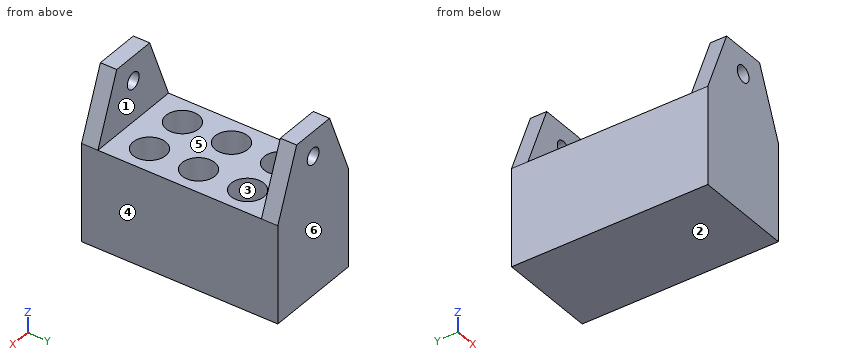
```python
from build123d import *

# Parameters (mm, degrees)
F0_W       = 38.1
F0_H       = 76.2
F0_R       = 6.35
F1_DEPTH   = 38.1
F2_DEPTH   = 12.7
F3_W       = 38.1
F3_H       = 6.35
F4_DEPTH   = 25.4
F5_SIZE2   = 10.16
F5_SIZE    = 25.4
F6_SIZE2   = 10.16
F6_SIZE    = 25.4
F6_2_SIZE2 = 10.16
F6_2_SIZE  = 25.4
F7_R       = 3.175
F8_DEPTH   = 105.84064


with BuildPart() as f1:
    # F0 (on Top) → F1 (new body)
    with BuildSketch(Plane.XY):
        with Locations((19.05, 38.1)):
            Rectangle(F0_W, F0_H)
        with Locations((10.16, 19.05)):
            Circle(F0_R, mode=Mode.SUBTRACT)
        with Locations((27.94, 19.05)):
            Circle(F0_R, mode=Mode.SUBTRACT)
        with Locations((10.16, 38.1)):
            Circle(F0_R, mode=Mode.SUBTRACT)
        with Locations((10.16, 57.15)):
            Circle(F0_R, mode=Mode.SUBTRACT)
        with Locations((27.94, 38.1)):
            Circle(F0_R, mode=Mode.SUBTRACT)
        with Locations((27.94, 57.15)):
            Circle(F0_R, mode=Mode.SUBTRACT)
    extrude(amount=F1_DEPTH)

    # F0 (on Top) → F2 (join)
    with BuildSketch(Plane.XY):
        with Locations((10.16, 57.15)):
            Circle(F0_R)
        with Locations((27.94, 57.15)):
            Circle(F0_R)
        with Locations((27.94, 38.1)):
            Circle(F0_R)
        with Locations((10.16, 19.05)):
            Circle(F0_R)
        with Locations((27.94, 19.05)):
            Circle(F0_R)
        with Locations((10.16, 38.1)):
            Circle(F0_R)
    extrude(amount=F2_DEPTH)

    # F3 (on face) → F4 (join)
    with BuildSketch(Plane.XY.offset(38.1)):
        with Locations((19.05, 73.025)):
            Rectangle(F3_W, F3_H)
        with Locations((19.05, 3.175)):
            Rectangle(F3_W, F3_H)
    extrude(amount=F4_DEPTH)

    # F5
    f5_edges = [f1.edges().sort_by_distance(p)[0] for p in [
        (38.1, 73.025, 63.5),
        (0, 73.025, 63.5),
    ]]
    chamfer(f5_edges, length=F5_SIZE, length2=F5_SIZE2)

    # F6
    f6_edges = [f1.edges().sort_by_distance(p)[0] for p in [
        (38.1, 3.175, 63.5),
    ]]
    f6_side = f1.faces().sort_by_distance((38.1, 36.261842, 20.721053))[0]
    chamfer(f6_edges, length=F6_SIZE, length2=F6_SIZE2, reference=f6_side)

    # F6#2
    f6_2_edges = [f1.edges().sort_by_distance(p)[0] for p in [
        (0, 3.175, 63.5),
    ]]
    f6_2_side = f1.faces().sort_by_distance((0, 36.261842, 20.721053))[0]
    chamfer(f6_2_edges, length=F6_2_SIZE, length2=F6_2_SIZE2, reference=f6_2_side)

    # F7 (on face) → F8 (cut)
    with BuildSketch(Plane(origin=(0, 76.2, 0), x_dir=(-1, 0, 0), z_dir=(0, 1, 0))):
        with Locations((-19.05, 53.975)):
            Circle(F7_R)
    extrude(amount=-F8_DEPTH, mode=Mode.SUBTRACT)


solid = f1.part
```
Work out the finished part from the listing and answer in its coordinate system (mm). Face numbers are marked on the shaded views. A direction names the side the tool comes from. Coordinates: 2 decimals unless noted, no trailing zeros. Write each loop counter-clockwise with the first axis right and the second up, starting at its lowest first coordinate (ties: lowest second). Pieces come first, ordered by that corner, then holes.
Q1. Determine the mould class of the marked faces 4, 5 and 6 for opening direction Y: released by +Y, released by -Y, zero draft, split by the parting line, or undercut.
Q2. Each of these flat-tipped pins is pushed along its axis until it touches: pin 1 Ø10 at (x, y) = (7.5, 37) entering from +Z; pin 2 Ø2 at (x, y) = (32, 40) entering from +Z. Where does it stop, or does it pass through?
Q3. A cutting plane is placed at D-D, the plane x = 14.5. Give the vertices of the cut face in (y, z).
Q4. Find the intervals of material crossed by line 1 (X direction, y = 57, z = 26); line 2 (Y direction, x = 27.94, z = 29.5); line 3 (Y direction, x = 18, z = 59), in increasing order.
Q5. A cutting plane is placed at C-C, the plane y = 19.05. Give the vertices of the cut face in (x, z).
Q6. Which of the six approach directions +Z, -Z, +X, -X, +Y, -Y give full straight-line access (tool end or side, diameter ignored) to the marked faces 1, 2 and 3?
Q7. A cutting plane is placed at B-B, the plane z = 33. Give the vertices of the cut face in (x, y), then the cut area to 3 significant figures.
Q8. A cutting plane is placed at A-A, the plane x = 19.05. Give the vertices of the cut face in (y, z).
Findings below:
1. face 4: zero draft
1. face 5: undercut
1. face 6: released by +Y
2. pin 1: stops at z = 38.1
2. pin 2: stops at z = 12.7
3. outline: (0, 0) - (76.2, 0) - (76.2, 63.5) - (69.85, 63.5) - (69.85, 38.1) - (61.79, 38.1) - (61.79, 12.7) - (52.51, 12.7) - (52.51, 38.1) - (42.74, 38.1) - (42.74, 12.7) - (33.46, 12.7) - (33.46, 38.1) - (23.69, 38.1) - (23.69, 12.7) - (14.41, 12.7) - (14.41, 38.1) - (6.35, 38.1) - (6.35, 63.5) - (0, 63.5) - close
4. line 1: x = 0 to 3.81, 16.51 to 21.59, 34.29 to 38.1
4. line 2: y = 0 to 12.7, 25.4 to 31.75, 44.45 to 50.8, 63.5 to 76.2
4. line 3: y = 0 to 6.35, 69.85 to 76.2
5. outline: (0, 0) - (38.1, 0) - (38.1, 38.1) - (34.29, 38.1) - (34.29, 12.7) - (21.59, 12.7) - (21.59, 38.1) - (16.51, 38.1) - (16.51, 12.7) - (3.81, 12.7) - (3.81, 38.1) - (0, 38.1) - close
6. face 1: +Z, +X, -X
6. face 2: -Z, +X, -X, +Y, -Y
6. face 3: +Z
7. outline: (0, 0) - (38.1, 0) - (38.1, 76.2) - (0, 76.2) - close; hole circle Ø12.7 at (10.16, 19.05); hole circle Ø12.7 at (10.16, 38.1); hole circle Ø12.7 at (10.16, 57.15); hole circle Ø12.7 at (27.94, 19.05); hole circle Ø12.7 at (27.94, 38.1); hole circle Ø12.7 at (27.94, 57.15)
7. area: 2,140 mm2
8. outline: (0, 0) - (76.2, 0) - (76.2, 50.8) - (69.85, 50.8) - (69.85, 38.1) - (6.35, 38.1) - (6.35, 50.8) - (0, 50.8) - close; (0, 57.15) - (6.35, 57.15) - (6.35, 63.5) - (0, 63.5) - close; (69.85, 57.15) - (76.2, 57.15) - (76.2, 63.5) - (69.85, 63.5) - close
